Check sheet for the drawn part. Datum: minimum x, y, z corner. Units: mm. A direction names the side the tool comes from. Round coordinates to 2 decimals unless told otherwise and drop trailing zeros. Write each loop counter-clockwise with the first axis right and the second up, starting at its lowest first coordinate (ties: lowest second). Pieces come first, ordered by that corner, then holes. Notation, with made-up numbers: M 10,76.5 L 42,76.5 A24 cw 42,88.5 Z; hole C 81.5,20 d3. An arc over 180 degrees is marked long. Answer in a Markdown table with one row per item. Add a question column.
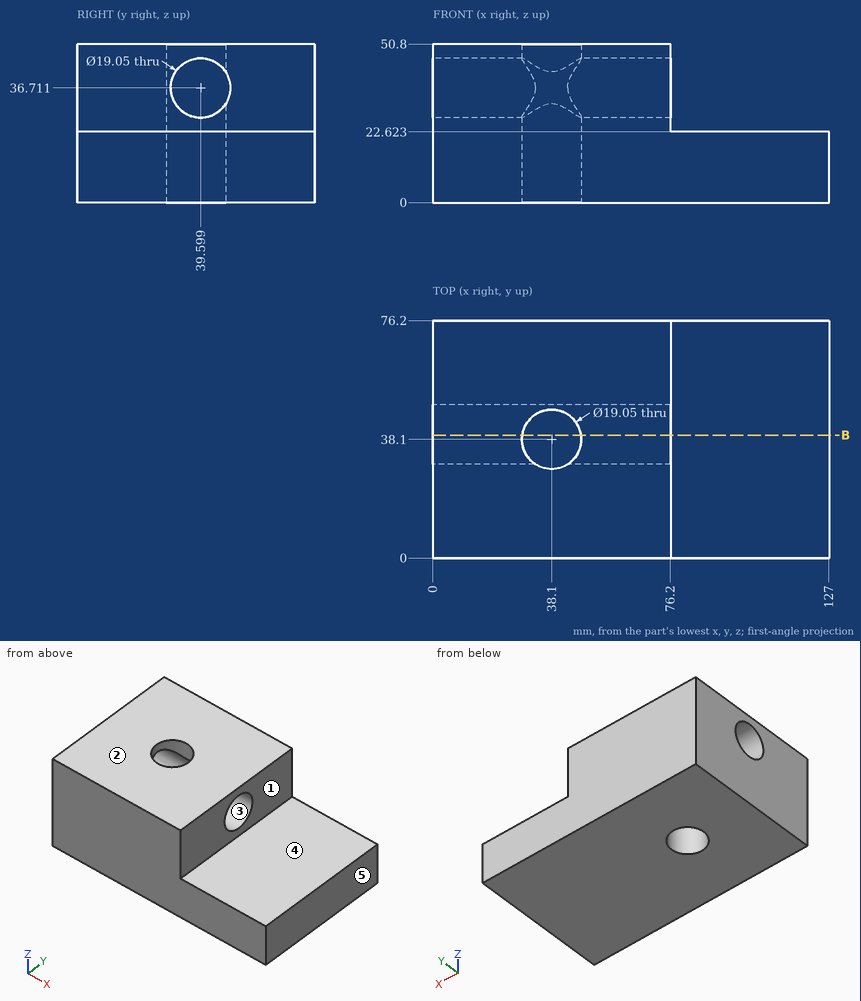
Item 1: Access from +Z, -Z, +X, -X, +Y, -Y to the whole of each face (thin tool, end or side, straight path). Record for the marked faces 4 and 5.
Item 2: Mould release check, pull along Z, two halves, no side actions. Record for the marked faces 1, 2 and 3: +Z half, -Z half, draft (parallel to the pull), parting line (faces both ways), or undercut.
Item 3: Section check B-B, the plane y = 39.5. Record the boundary of the cut face in (x, z) (1 decimal).
Item 4: Scan lines: probe 1 along Y at (x, z) = (38, 18) (1 decimal); probe 2 along Z at (x, y) = (99, 39.5). Record each from-to range of solid material in increasing order. Write a range as from..to.
Item 5: Gauge pin test, flat ends, axial feed: pin 1 Ø4 at (x, y) = (100, 68) entering from +Z; pin 2 Ø2 at (y, z) = (59.5, 42.5) entering from +X. Record the tip position at first contact, or that the pin passes through.
Result sheet:
| question | item | result |
|---|---|---|
| 1 | face 4 | +Z, +X, +Y, -Y |
| 1 | face 5 | +Z, -Z, +X, +Y, -Y |
| 2 | face 1 | draft |
| 2 | face 2 | +Z half |
| 2 | face 3 | undercut |
| 3 | outline | M 0,0 L 28.7,0 L 28.7,27.2 L 0,27.2 Z; M 0,46.2 L 28.7,46.2 L 28.7,50.8 L 0,50.8 Z; M 47.5,0 L 127,0 L 127,22.6 L 76.2,22.6 L 76.2,27.2 L 47.5,27.2 Z; M 47.5,46.2 L 76.2,46.2 L 76.2,50.8 L 47.5,50.8 Z |
| 4 | probe 1 | y = 0..28.6, 47.6..76.2 |
| 4 | probe 2 | z = 0..22.62 |
| 5 | pin 1 | stops at z = 22.62 |
| 5 | pin 2 | stops at x = 76.2 |
